Autodesk Inventor part; units mm, degrees
ref_plane "YZ Plane" through (0, 0, 0) normal (1, 0, 0) x (0, 1, 0)
ref_plane "XZ Plane" through (0, 0, 0) normal (0, 1, 0) x (-1, 0, 0)
ref_plane "XY Plane" through (0, 0, 0) normal (0, 0, 1) x (1, 0, 0)
sketch "Boceto1" plane through (0, 0, 0) normal (0, 1, 0) x (-1, 0, 0)
  line L0 (11.708, 26.8389) -> (11.708, -1.1611)
  line L1 (11.708, -1.1611) -> (-39.292, -1.1611)
  line L2 (-39.292, -1.1611) -> (-39.292, 26.8389)
  line L3 (-39.292, 26.8389) -> (11.708, 26.8389)
  circle A0 centre (4.833, 13.4639) radius 2
  circle A1 centre (-32.417, 13.4639) radius 2
  circle A2 centre (-13.792, 18.6686) radius 2
  point P0 (0, 0)
  point P1 (0, 0)
  dimension "d0" = 28
  dimension "d1" = 51
  dimension "d2" = 4
  dimension "d3" = 4
  dimension "d4" = 4
  dimension "d5" = 25.5
  dimension "d6" = 6.875
  dimension "d7" = 13.375
  dimension "d8" = 6.875
  dimension "d9" = 13.375
extrude "Extrusión1" add sketch "Boceto1" along normal blind 1
sketch "Boceto2" plane through (39.292, 0, 26.8389) normal (1, 0, 0) x (0, 0, -1)
  arc A0 (30.75, 0) -> (28, 2.75) centre (30.75, 2.75) ccw
  circle A1 centre (30.75, 2.75) radius 1.875
  line L0 (0, 0) -> (28, 0)
  line L1 (28, 0) -> (28, 1)
  line L2 (28, 0) -> (30.75, 0)
  line L3 (28, 0) -> (28, 2.75)
  point P0 (26.8389, 0)
  dimension "d12" = 5.5
  dimension "d13" = 3.75
extrude "Extrusión2" add sketch "Boceto2" against normal blind 38
sketch "Boceto3" plane through (39.292, 0, 26.8389) normal (1, 0, 0) x (0, 0, -1)
  circle A0 centre (30.75, 2.75) radius 1.875
  arc A1 (30.75, 0) -> (28, 2.75) centre (30.75, 2.75) ccw
  arc A2 (30.75, 0) -> (28, 2.75) centre (30.75, 2.75) ccw
  line L0 (28, 2.75) -> (28, 0)
  line L1 (28, 0) -> (30.75, 0)
  point P0 (26.8389, 0)
extrude "Extrusión3" cut sketch "Boceto3" against normal blind 13
properties part number "Ala 2 Bisagra tipo Libro Grande"
The model under review builds one solid part; all positions refer to its coordinate system, in mm. A direction names the side the tool comes from. Coordinates: 2 decimals unless noted, no trailing zeros. Write each loop counter-clockwise with the first axis right and the second up, starting at its lowest first coordinate (ties: lowest second). Pieces come first, ordered by that corner, then holes. Notation, with made-up numbers: (7, 27.25) -> (34, 27.25) arc R12 ccw to (34, 32.25) -> close; hole circle Ø6 at (13, 15.5). An arc over 180 degrees is marked (long way). Answer in a Markdown table with one row per item.
1. We need section B-B, the plane x = 22. State the section outline as (y, z) points (3 decimals).
Answers below:
| item | result |
|---|---|
| outline | (0, -3.911) arc R2.75 ccw (long way) to (2.75, -1.161) -> (1, -1.161) -> (1, 26.839) -> (0, 26.839) -> close; hole circle Ø3.75 at (2.75, -3.911) |
2. Clearance check with flat-ended pins moving along their axes: pin 1 Ø3 at (y, z) = (1.5, 4) entering from -X; pin 2 Ø3 at (y, z) = (2.5, -3.5) entering from -X; pin 3 Ø1.4 at (x, y) = (15, 2) entering from +Z; pin 4 Ø4 at (x, z) = (6, 20) entering from +Y. State where each tip first meets the part, or that it passes through.
Answers below:
| item | result |
|---|---|
| pin 1 | stops at x = -11.71 |
| pin 2 | stops at x = 1.29 |
| pin 3 | stops at z = -1.16 |
| pin 4 | stops at y = 1 |
3. For faces 1 (the flat face through (32.9, 0.5, -1.161)), 2 (the flat face through (1.292, 2, -2)), 3 (the flat face through (14, 1, 13)), list the 3-axis set-ups (+Z, -Z, +X, -X, +Y, -Y) from which the entire face can be reached by the end or side of a thin tool; tool diameter is ignored.
Answers below:
| item | result |
|---|---|
| face 1 | -Z, +X, +Y, -Y |
| face 2 | -Z, -X, +Y, -Y |
| face 3 | +Z, +X, -X, +Y |
4. We need section C-C, the plane x = -5.5. State the section outline as (y, z) points.
Answers below:
| item | result |
|---|---|
| outline | (0, -1.16) -> (1, -1.16) -> (1, 11.58) -> (0, 11.58) -> close; (0, 15.35) -> (1, 15.35) -> (1, 26.84) -> (0, 26.84) -> close |
5. Wall thickness on probe 1 along Y at (x, z) = (13, 3); probe 2 along Z at (x, y) = (16, 1.1); probe 3 along Z at (x, y) = (22, 0.5): over which ranges is each line inside the solid? List them lowest first. Write a range as [from, to].
Answers below:
| item | result |
|---|---|
| probe 1 | y = [0, 1] |
| probe 2 | z = [-6.11, -4.8], [-3.02, -1.16] |
| probe 3 | z = [-5.49, 26.84] |
6. We need section D-D, the plane z = 24. State the section outline as (x, y) points.
Answers below:
| item | result |
|---|---|
| outline | (-11.71, 0) -> (39.29, 0) -> (39.29, 1) -> (-11.71, 1) -> close |
7. We need section A-A, the plane y = 3.75. State the section outline as (x, z) points.
Answers below:
| item | result |
|---|---|
| outline | (1.29, -6.47) -> (26.29, -6.47) -> (26.29, -5.5) -> (1.29, -5.5) -> close; (1.29, -2.33) -> (26.29, -2.33) -> (26.29, -1.35) -> (1.29, -1.35) -> close |
8. Draft analysis for pull direction Z (two halves, no side actions). For faces 4 (the cylindrical face through (-4.57, 0.49, 11.48)), 5 (the flat face through (14, 2, -1.161)), 6 (the cylindrical face through (11.945, 0.493, 19.435)), 7 (the flat face through (-5.3, 0.5, -1.161)), state which applies: +Z half, -Z half, draft (parallel to the pull), parting line (faces both ways), or undercut.
Answers below:
| item | result |
|---|---|
| face 4 | undercut |
| face 5 | +Z half |
| face 6 | undercut |
| face 7 | -Z half |
